Can you work these out from the model? Positions are in its coordinate system, mm. A direction names the side the tool comes from. Round coordinates to 2 decimals unless told otherwise and drop trailing zeros. Order: outer loops, then holes, each group sorted by start corner. A loop starts at its lowest first (then second) coordinate and runs counter-clockwise, first axis right, second up. Notation, with made-up numbers: (56.5, 17.5) -> (63.5, 17.5) arc R18 ccw to (63.5, 41.5) -> close; hole circle Ø4 at (42.5, 78.25). An arc over 180 degrees is marked (long way). One line per item, written item: value.
```python
from build123d import *

# Parameters (mm, degrees)
CYLINDER002_R     = 1
CYLINDER002_DEPTH = 5
CYLINDER003_R     = 1
CYLINDER003_DEPTH = 5
CYLINDER004_R     = 1
CYLINDER004_DEPTH = 5
CYLINDER005_R     = 1.25
CYLINDER005_DEPTH = 50
CYLINDER001_R     = 1
CYLINDER001_DEPTH = 5
CYLINDER_R        = 7.5
CYLINDER_DEPTH    = 1.5
CYLINDER006_R     = 2.5
CYLINDER006_DEPTH = 50
BOX_W             = 20
BOX_H             = 30
BOX_DEPTH         = 20


with BuildPart() as cylinder002:
    # Cylinder002 → Cylinder002 (new body)
    with BuildSketch(Plane(origin=(-8, 0, 8), x_dir=(1, 0, 0), z_dir=(0, 1, 0))):
        Circle(CYLINDER002_R)
    extrude(amount=CYLINDER002_DEPTH)


with BuildPart() as cylinder003:
    # Cylinder003 → Cylinder003 (new body)
    with BuildSketch(Plane(origin=(8, 0, -8), x_dir=(1, 0, 0), z_dir=(0, 1, 0))):
        Circle(CYLINDER003_R)
    extrude(amount=CYLINDER003_DEPTH)


with BuildPart() as cylinder004:
    # Cylinder004 → Cylinder004 (new body)
    with BuildSketch(Plane(origin=(8, 0, 8), x_dir=(1, 0, 0), z_dir=(0, 1, 0))):
        Circle(CYLINDER004_R)
    extrude(amount=CYLINDER004_DEPTH)


with BuildPart() as cylinder005:
    # Cylinder005 → Cylinder005 (new body)
    with BuildSketch(Plane(origin=(0, -12, 0), x_dir=(1, 0, 0), z_dir=(0, 1, 0))):
        Circle(CYLINDER005_R)
    extrude(amount=CYLINDER005_DEPTH)


with BuildPart() as fusion002:
    # Cylinder001 → Cylinder001 (new body)
    with BuildSketch(Plane(origin=(-8, 0, -8), x_dir=(1, 0, 0), z_dir=(0, 1, 0))):
        Circle(CYLINDER001_R)
    extrude(amount=CYLINDER001_DEPTH)

    # Fusion002: union Cylinder002, Cylinder003, Cylinder004, Cylinder005
    add(cylinder002.part)
    add(cylinder003.part)
    add(cylinder004.part)
    add(cylinder005.part)


with BuildPart() as cylinder:
    # Cylinder → Cylinder (new body)
    with BuildSketch(Plane(origin=(0, -1.5, 0), x_dir=(1, 0, 0), z_dir=(0, 1, 0))):
        Circle(CYLINDER_R)
    extrude(amount=CYLINDER_DEPTH)


with BuildPart() as cylinder006:
    # Cylinder006 → Cylinder006 (new body)
    with BuildSketch(Plane(origin=(0, -12, 0), x_dir=(1, 0, 0), z_dir=(0, 1, 0))):
        Circle(CYLINDER006_R)
    extrude(amount=CYLINDER006_DEPTH)


with BuildPart() as hollowdoubleshaftstepper:
    # Box → Box (new body)
    with BuildSketch(Plane(origin=(-10, 0, -10), x_dir=(1, 0, 0), z_dir=(0, 0, 1))):
        with Locations((10, 15)):
            Rectangle(BOX_W, BOX_H)
    extrude(amount=BOX_DEPTH)

    # Fusion001: union Cylinder, Cylinder006
    add(cylinder.part)
    add(cylinder006.part)

    # Cut: cut Fusion002
    add(fusion002.part, mode=Mode.SUBTRACT)


solid = hollowdoubleshaftstepper.part
```
Q1. We'd pull the mould along Z, two halves only. Please class faces 1 (the face through (-10, 15, 0)), 2 (the face through (0, 15, 10)), 3 (the face through (-8, 2, -9)): released by +Z, released by -Z, zero draft, split by the parting line, or undercut.
Answers below:
face 1: zero draft
face 2: released by +Z
face 3: undercut
Q2. I want a section at D-D on z = 8. List the corners of the cut face in (x, y) for me, plus the area to 3 significant figures.
Answers below:
outline: (-10, 0) -> (-9, 0) -> (-9, 5) -> (-7, 5) -> (-7, 0) -> (7, 0) -> (7, 5) -> (9, 5) -> (9, 0) -> (10, 0) -> (10, 30) -> (-10, 30) -> close
area: 580 mm^2
Q3. Will these pins go through, and if not, where does the flat tip stop? pin 1 Ø4 at (y, z) = (-4, -1) entering from +X; pin 2 Ø4 at (x, z) = (-2, 2.5) entering from +Y; pin 3 Ø0.6 at (x, z) = (-8.5, -8) entering from -Y; pin 4 Ø3 at (x, z) = (-8, 8) entering from -Y.
Answers below:
pin 1: x = 2.5
pin 2: y = 38
pin 3: y = 5
pin 4: y = 0
Q4. Please list where these lines run through material, in increasing order: line 1 along X through (y, z) = (1.45, -8); line 2 along Y through (x, z) = (-8.5, 1.25).
Answers below:
line 1: -10 to -9, -7 to 7, 9 to 10
line 2: 0 to 30
Q5. I want a section at B-B on z = 0. List the corners of the cut face in (x, y) for me, plus the area to 3 significant figures.
Answers below:
outline: (-10, 0) -> (-7.5, 0) -> (-7.5, -1.5) -> (-2.5, -1.5) -> (-2.5, -12) -> (-1.25, -12) -> (-1.25, 38) -> (-2.5, 38) -> (-2.5, 30) -> (-10, 30) -> close; (1.25, -12) -> (2.5, -12) -> (2.5, -1.5) -> (7.5, -1.5) -> (7.5, 0) -> (10, 0) -> (10, 30) -> (2.5, 30) -> (2.5, 38) -> (1.25, 38) -> close
area: 590 mm^2
Q6. On a 3-axis mill with a long thin cutter (end or side, diameter ignored), from which of +Z, -Z, +X, -X, +Y, -Y can I reach the whole of each face in a straight line? I mean faces 4 (the face through (-2, 30, 2)), 5 (the face through (10, 15, 0)), 6 (the face through (-8, 5, -8)). Say none if no direction works.
Answers below:
face 4: +Y
face 5: +Z, -Z, +X, +Y, -Y
face 6: -Y
Q7. I want a section at A-A on x = 0. List the corners of the cut face in (y, z) for me, plus the area to 3 significant figures.
Answers below:
outline: (-12, -2.5) -> (-1.5, -2.5) -> (-1.5, -7.5) -> (0, -7.5) -> (0, -10) -> (30, -10) -> (30, -2.5) -> (38, -2.5) -> (38, -1.25) -> (-12, -1.25) -> close; (-12, 1.25) -> (38, 1.25) -> (38, 2.5) -> (30, 2.5) -> (30, 10) -> (0, 10) -> (0, 7.5) -> (-1.5, 7.5) -> (-1.5, 2.5) -> (-12, 2.5) -> close
area: 590 mm^2
Q8. I want a section at C-C on y = 0.5. List the corners of the cut face in (x, z) for me.
Answers below:
outline: (-10, -10) -> (10, -10) -> (10, 10) -> (-10, 10) -> close; hole circle Ø2 at (-8, -8); hole circle Ø2 at (-8, 8); hole circle Ø2.5 at (0, 0); hole circle Ø2 at (8, -8); hole circle Ø2 at (8, 8)
